Part model, mm, in its own coordinate system. A direction names the side the tool comes from. Give positions to 0.01 mm unless a question says otherwise; leave off trailing zeros. Write each loop counter-clockwise with the first axis right and the second up, starting at its lowest first coordinate (ties: lowest second). Pieces come first, ordered by that corner, then holes. Notation, with made-up numbers: M 83.25,23 L 114.25,23 A33 ccw 114.25,54 Z; hole C -3,53.5 d6. An arc over 180 degrees is marked long. Use a Markdown table: item, result.
```python
from build123d import *

# Parameters (mm, degrees)
SKETCH_1_W          = 70
SKETCH_1_H          = 30
SKETCH_1_R          = 3.3
EXTRUDE_1_DEPTH     = 5
SKETCH_2_W          = 30
SKETCH_2_H          = 30
EXTRUDE_2_DEPTH     = 20
SKETCH_3_R          = 13
CUT_EXTRUDE_1_DEPTH = 26
EXTRUDE_3_DEPTH     = 4


with BuildPart() as part:
    # 草图1 → 凸台-拉伸1 (new body)
    with BuildSketch(Plane.XY):
        Rectangle(SKETCH_1_W, SKETCH_1_H)
        with Locations((-28, 0)):
            Circle(SKETCH_1_R, mode=Mode.SUBTRACT)
        with Locations((28, 0)):
            Circle(SKETCH_1_R, mode=Mode.SUBTRACT)
    extrude(amount=EXTRUDE_1_DEPTH)

    # 草图2 → 凸台-拉伸2 (add)
    with BuildSketch(Plane.XY.offset(5)):
        Rectangle(SKETCH_2_W, SKETCH_2_H)
    extrude(amount=EXTRUDE_2_DEPTH)

    # 草图3 → 切除-拉伸1 (cut, through all)
    with BuildSketch(Plane.XY.offset(25)):
        Circle(SKETCH_3_R)
    extrude(amount=-CUT_EXTRUDE_1_DEPTH, mode=Mode.SUBTRACT)

    # 草图5 → 凸台-拉伸3 (add)
    with BuildSketch(Plane.XZ.offset(15)):
        Polygon((-35, 5), (-15, 25), (-15, 5), align=None)
        Polygon((15, 25), (35, 5), (15, 5), align=None)
    extrude_3 = extrude(amount=-EXTRUDE_3_DEPTH)

    # 镜向1: 凸台-拉伸3 across plane
    add(extrude_3.mirror(Plane.ZX))


solid = part.part
```
1. Drill centre lines: L1, parallel to Y at x = 28, z = 1.8; L2, parallel to Z at x = 24, y = -1.5; L3, parallel to Y at x = 2, z = 1.5. Where is each one in solid material? Low to high.
Findings below:
| item | result |
|---|---|
| L1 | -15 to -3.3, 3.3 to 15 |
| L2 | 0 to 5 |
| L3 | -15 to -12.85, 12.85 to 15 |
2. Cut at C-C, the plane x = 0. Give the cut face in (y, z), then the cut area to 3 significant figures.
Findings below:
| item | result |
|---|---|
| outline | M -15,0 L -13,0 L -13,25 L -15,25 Z; M 13,0 L 15,0 L 15,25 L 13,25 Z |
| area | 100 mm2 |
3. Cut at D-D, the plane z = 2.25. Give the cut face in (x, y), then the cut area to 3 significant figures.
Findings below:
| item | result |
|---|---|
| outline | M -35,-15 L 35,-15 L 35,15 L -35,15 Z; hole C -28,0 d6.6; hole C 0,0 d26; hole C 28,0 d6.6 |
| area | 1,500 mm2 |
4. Cut at B-B, the plane y = 5. Give the cut face in (x, z).
Findings below:
| item | result |
|---|---|
| outline | M -35,0 L -12,0 L -12,25 L -15,25 L -15,5 L -35,5 Z; M 12,0 L 35,0 L 35,5 L 15,5 L 15,25 L 12,25 Z |
5. Drop flat-ended pins along their axis: P1, Ø3, axis at x = 10.5, y = 0, coming from the -Z side; P2, Ø6, axis at x = 29, y = 3.5, coming from the +Z side. Give the stop position or say it passes through.
Findings below:
| item | result |
|---|---|
| P1 | through |
| P2 | z = 5 |
6. Cut at A-A, the plane z = 19.5. Give the cut face in (x, y), then the cut area to 3 significant figures.
Findings below:
| item | result |
|---|---|
| outline | M -20.5,-15 L 20.5,-15 L 20.5,-11 L 15,-11 L 15,11 L 20.5,11 L 20.5,15 L -20.5,15 L -20.5,11 L -15,11 L -15,-11 L -20.5,-11 Z; hole C 0,0 d26 |
| area | 457 mm2 |
7. Two-plate mould, pull along Y, no slides. Class faces 4 (the flat face through (35, 0, 2)), 5 (the flat face through (15, 0, 15)), 6 (the flat face through (0, -15, 10)): released by +Y, released by -Y, zero draft, split by the parting line, or undercut.
Findings below:
| item | result |
|---|---|
| face 4 | zero draft |
| face 5 | undercut |
| face 6 | released by -Y |
8. Tool access for faces 1 (the flat face through (-20, -11, 11)), 2 (the cylindrical face through (31.05, -1.26, 2.46)), 3 (the flat face through (21, 11, 11)): list every direction of +Z, -Z, +X, -X, +Y, -Y with a clear straight run to the whole face (end or side of a thin tool).
Findings below:
| item | result |
|---|---|
| face 1 | +Z, -X |
| face 2 | +Z, -Z |
| face 3 | +Z, +X |
